Part model, mm, in its own coordinate system. A direction names the side the tool comes from. Coordinates: 2 decimals unless noted, no trailing zeros. Order: outer loops, then holes, each group sorted by start corner. A loop starts at its lowest first (then second) coordinate and runs counter-clockwise, first axis right, second up.
```python
from build123d import *

# Parameters (mm, degrees)
SKETCH1_R           = 5.2
SKETCH1_R_2         = 1.4
BOSS_EXTRUDE1_DEPTH = 10
SKETCH2_W           = 124
SKETCH2_H           = 5
CUT_EXTRUDE1_DEPTH  = 158.353106102
FILLET1_R           = 5
SKETCH3_W           = 8
SKETCH3_H           = 32
BOSS_EXTRUDE2_DEPTH = 5
SKETCH4_R           = 1.4
CUT_EXTRUDE2_DEPTH  = 162.124175716


with BuildPart() as part:
    # Sketch1 → Boss-Extrude1 (new body)
    with BuildSketch(Plane(origin=(0, 0, 0), x_dir=(1, 0, 0), z_dir=(0, 1, 0))):
        Polygon((0, 0), (16, 0), (16, 5), (140, 5), (140, 0), (156, 0), (156, 18), (140, 18), (140, 13), (16, 13), (16, 18), (0, 18), align=None)
        with Locations(Location((8, 9, 0), (0, 0, 270))):
            Circle(SKETCH1_R, mode=Mode.SUBTRACT)
        with Locations(Location((148, 9, 0), (0, 0, 270))):
            Circle(SKETCH1_R, mode=Mode.SUBTRACT)
        with Locations(Location((28, 9, 0), (0, 0, 270))):
            Circle(SKETCH1_R_2, mode=Mode.SUBTRACT)
        with Locations(Location((128, 9, 0), (0, 0, 90))):
            Circle(SKETCH1_R_2, mode=Mode.SUBTRACT)
    extrude(amount=BOSS_EXTRUDE1_DEPTH)

    # Sketch2 → Cut-Extrude1 (cut, through all)
    with BuildSketch(Plane.XY):
        with Locations((78, 7.5)):
            Rectangle(SKETCH2_W, SKETCH2_H)
    extrude(amount=-CUT_EXTRUDE1_DEPTH, mode=Mode.SUBTRACT)

    # Fillet1
    fillet1_edges = [part.edges().sort_by_distance(p)[0] for p in [
        (140, 5, 0),
        (156, 5, 0),
        (156, 5, -18),
        (140, 5, -18),
        (0, 5, 0),
        (0, 5, -18),
        (16, 5, -18),
        (16, 5, 0),
    ]]
    fillet(fillet1_edges, radius=FILLET1_R - 0.0001)  # a hair under: the kernel refuses the full size


with BuildPart() as body_2:
    # Body-Move/Copy1: copy of part
    add(part.part.moved(Location((0, 0, 40))))


with BuildPart() as part_1:
    add(part.part)

    add(body_2.part)  # Boss-Extrude2 merges body 2
    # Sketch3 → Boss-Extrude2 (add)
    with BuildSketch(Plane(origin=(0, 0, 0), x_dir=(1, 0, 0), z_dir=(0, 1, 0))):
        with Locations((53, -11)):
            Rectangle(SKETCH3_W, SKETCH3_H)
        with Locations((103, -11)):
            Rectangle(SKETCH3_W, SKETCH3_H)
    extrude(amount=BOSS_EXTRUDE2_DEPTH)

    # Sketch4 → Cut-Extrude2 (cut, through all)
    with BuildSketch(Plane(origin=(0, 5, 0), x_dir=(1, 0, 0), z_dir=(0, 1, 0))):
        with Locations(Location((53, -11, 0), (0, 0, 270))):
            Circle(SKETCH4_R)
        with Locations(Location((103, -11, 0), (0, 0, 270))):
            Circle(SKETCH4_R)
    extrude(amount=-CUT_EXTRUDE2_DEPTH, mode=Mode.SUBTRACT)


solid = part_1.part
```
(1) Tool access for faces 1 (the face through (107, 2, 11)), 2 (the face through (140, 7, 31)), 3 (the face through (14, 5, -17)): list every direction of +Z, -Z, +X, -X, +Y, -Y with a clear straight run to the whole face (end or side of a thin tool).
(2) Pull direction Z, two halves, no side cores. Call faces 4 (the face through (153.156, 4.93, -9.677)), 5 (the face through (142, 5, -17)), 6 (the face through (14, 5, -1)), 7 (the face through (77.1, 5, 27.3)): +Z half, -Z half, draft (parallel to the pull), parting line (faces both ways), or undercut.
(3) Slice it at B-B, the plane x = 53. Give the cut face in (y, z).
(4) Probe line 1 (X direction, y = 4, z = 31); line 2 (Z direction, x = 128, y = 1.15); line 3 (X direction, y = 3.75, z = 11). List the from-to ranges inside material, lowest first.
(5) Slice it at A-A, the plane z = 5. Give the cut face in (x, y), then the cut area to 3 significant figures.
(6) Slice it at C-C, the plane x = 128. Give the cut face in (y, z), then the cut area to 3 significant figures.
(7) Slice it at D-D, the plane y = 7.25. State how many separate pieces and enclosed holes the cut face has, then the cut area to 3 significant figures.
(8) Drop flat-ended pins along their axis: pin 1 (12 mm diameter, centred on x = 98.5, z = 11, fed in from +Y); pin 2 (2.5 mm diameter, centred on y = 3, z = 14, fed in from +X); pin 3 (4 mm diameter, centred on x = 81.5, y = 1.5, fed in from +Z). Give the stop position or say it passes through.
Here are the results:
1. face 1: +Y, -Y
1. face 2: +Z, -Z, +Y
1. face 3: -Z, +Y, -Y
2. face 4: undercut
2. face 5: -Z half
2. face 6: undercut
2. face 7: draft
3. outline: (0, -13) - (5, -13) - (5, 9.6) - (0, 9.6) - close; (0, 12.4) - (5, 12.4) - (5, 35) - (0, 35) - close
4. line 1: x = 0 to 2.8, 13.2 to 26.6, 29.4 to 126.6, 129.4 to 142.8, 153.2 to 156
4. line 2: z = -13 to -10.4, -7.6 to -5, 27 to 29.6, 32.4 to 35
4. line 3: x = 49 to 51.6, 54.4 to 57, 99 to 101.6, 104.4 to 107
5. outline: (49, 0) - (57, 0) - (57, 5) - (49, 5) - close; (99, 0) - (107, 0) - (107, 5) - (99, 5) - close
5. area: 80.0 mm2
6. outline: (0, -13) - (5, -13) - (5, -10.4) - (0, -10.4) - close; (0, -7.6) - (5, -7.6) - (5, -5) - (0, -5) - close; (0, 27) - (5, 27) - (5, 29.6) - (0, 29.6) - close; (0, 32.4) - (5, 32.4) - (5, 35) - (0, 35) - close
6. area: 52.0 mm2
7. separate pieces: 4
7. enclosed holes: 4
7. area: 726 mm2
8. pin 1: stops at y = 5
8. pin 2: stops at x = 107
8. pin 3: stops at z = 35
